```python
from build123d import *

# Parameters (mm, degrees)
SKETCH1_R           = 1.75
BOSS_EXTRUDE1_DEPTH = 8.5
BOSS_EXTRUDE2_DEPTH = 8.5
CUT_EXTRUDE1_DEPTH  = 8.5
FILLET1_R           = 0.1


with BuildPart() as part:
    # Sketch1 → Boss-Extrude1 (new body)
    with BuildSketch(Plane(origin=(0, 0, 0), x_dir=(1, 0, 0), z_dir=(0, 1, 0))):
        with BuildLine():
            Line((0, 5), (22, 5))
            ThreePointArc((22, 5), (27, 0), (22, -5))
            Line((22, -5), (0, -5))
            ThreePointArc((0, -5), (-5, 0), (0, 5))
        make_face()
        with Locations(Location((0, 0, 0), (0, 0, 270))):
            Circle(SKETCH1_R, mode=Mode.SUBTRACT)
        with Locations(Location((22, 0, 0), (0, 0, 270))):
            Circle(SKETCH1_R, mode=Mode.SUBTRACT)
    extrude(amount=BOSS_EXTRUDE1_DEPTH)

    # Sketch2 → Boss-Extrude2 (add)
    with BuildSketch(Plane(origin=(0, 8.5, 0), x_dir=(1, 0, 0), z_dir=(0, 1, 0))):
        with BuildLine():
            Line((24.179012082, -4.476059884), (33.341557569, -0.026966843))
            add(Edge.make_bspline(
                [(33.341557569, -0.026966843), (41.749820473, 7.89313442), (52.969012082, 6.083442161)],
                knots=[0, 0, 0, 1, 1, 1], degree=2))
            Line((52.969012082, 6.083442161), (60.334686591, 9.205434959))
            Line((60.334686591, 9.205434959), (58.773690192, 12.888272213))
            add(Edge.make_bspline(
                [(58.773690192, 12.888272213), (52.774224243, 15.890799399), (35.603615653, 14.597846237), (21.152761079, 6.296000311), (11, 5)],
                knots=[0, 0, 0, 0, 0.392136184, 1, 1, 1, 1], degree=3))
            Line((11, 5), (22, 5))
            ThreePointArc((22, 5), (26.8616817, 1.129378711), (24.179012082, -4.476059884))
        make_face()
    extrude(amount=-BOSS_EXTRUDE2_DEPTH)

    # Sketch3 → Cut-Extrude1 (cut)
    with BuildSketch(Plane(origin=(0, 8.5, 0), x_dir=(1, 0, 0), z_dir=(0, 1, 0))):
        Polygon((53.093613314, 7.319249743), (52.969012082, 6.083442161), (54.158655304, 6.587680784), align=None)
        Polygon((54.199304069, 7.787904524), (54.158655304, 6.587680784), (55.255605115, 7.052630654), align=None)
        Polygon((55.31150405, 8.259318286), (55.255605115, 7.052630654), (56.367805096, 7.524044416), align=None)
        Polygon((56.423704031, 8.730732048), (56.367805096, 7.524044416), (57.480005077, 7.995458178), align=None)
        Polygon((57.535904012, 9.202145811), (57.480005077, 7.995458178), (58.592205058, 8.46687194), align=None)
        Polygon((58.648103993, 9.673559573), (58.592205058, 8.46687194), (59.704405039, 8.938285702), align=None)
        Polygon((59.909629601, 10.208266049), (59.704405039, 8.938285702), (60.334686591, 9.205434959), align=None)
    extrude(amount=-CUT_EXTRUDE1_DEPTH, mode=Mode.SUBTRACT)

    # Fillet1
    fillet1_edges = [part.edges().sort_by_distance(p)[0] for p in [
        (57.480005077, 4.25, -7.995458178),
        (59.704405039, 4.25, -8.938285702),
        (52.969012082, 4.25, -6.083442161),
        (54.158655304, 4.25, -6.587680784),
        (56.367805096, 4.25, -7.524044416),
        (58.592205058, 4.25, -8.46687194),
        (55.255605115, 4.25, -7.052630654),
    ]]
    fillet(fillet1_edges, radius=FILLET1_R)


solid = part.part
```
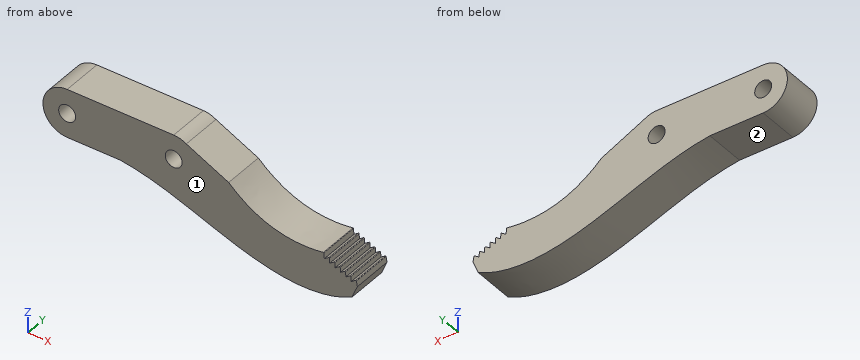
For this review, take the finished solid that the model builds, in its own axes (mm). Face numbers are marked on the shaded views. A direction names the side the tool comes from. Round coordinates to 2 decimals unless told otherwise and drop trailing zeros. Write each loop counter-clockwise with the first axis right and the second up, starting at its lowest first coordinate (ties: lowest second). Pieces come first, ordered by that corner, then holes. Notation, with made-up numbers: (42.25, 13.5) - (61.25, 13.5) arc R30 cw to (61.25, 35.5) - close; hole circle Ø11 at (76, 40.5). An arc over 180 degrees is marked (long way). Answer as a JSON object with one key per item and string values.
1. To check wall thickness, follow line 1 along X through (y, z) = (3.75, 0); line 2 along X through (y, z) = (3.5, 0.5); line 3 along Z through (x, y) = (3, 3.5). State the ranges of each line that lie inside material, in increasing order.
Response values:
{"line 1": "x = -5 to -1.75, 1.75 to 20.25, 23.75 to 33.37", "line 2": "x = -4.97 to -1.68, 1.68 to 20.32, 23.68 to 32.37", "line 3": "z = -5 to 5"}
2. We need section A-A on x = 3. Give the boundary of the cut face in (y, z), then the cut area to 3 significant figures.
Response values:
{"outline": "(0, -5) - (8.5, -5) - (8.5, 5) - (0, 5) - close", "area": "85.0 mm2"}
3. We need section B-B on z = -0.75. Count the separate pieces of the cut face and the enclosed holes in it, then the cut area to 3 significant figures.
Response values:
{"separate pieces": "3", "enclosed holes": "0", "area": "279 mm2"}
4. Tool access review of the marked faces 1 and 2: name each direction out of +Z, -Z, +X, -X, +Y, -Y from which nothing blocks a thin tool from reaching the whole face with its end or side.
Response values:
{"face 1": "+Z, -Z, +X, -X, -Y", "face 2": "-Z, -X, +Y, -Y"}
5. For pin 1 Ø4 at (y, z) = (1.5, 2.5) entering from +X; pin 2 Ø2.5 at (x, y) = (3.5, 5.5) entering from -Z, all flat-tipped, find the tip position at first contact; note any pin that passes through.
Response values:
{"pin 1": "stops at x = 32.37", "pin 2": "stops at z = -5"}
